from build123d import *

# Parameters (mm, degrees)
SKETCH1_R           = 21
SKETCH1_R_2         = 6
BOSS_EXTRUDE1_DEPTH = 1
SKETCH2_R           = 21
SKETCH2_R_2         = 2.7
SKETCH2_R_3         = 6
BOSS_EXTRUDE2_DEPTH = 5
SKETCH3_R           = 1.3
CUT_EXTRUDE1_DEPTH  = 4


with BuildPart() as part:
    # Sketch1 → Boss-Extrude1 (new body)
    with BuildSketch(Plane(origin=(0, 0, 0), x_dir=(1, 0, 0), z_dir=(0, 1, 0))):
        with Locations(Location((0, 0, 0), (0, 0, 270))):
            Circle(SKETCH1_R)
        with Locations(Location((0, 0, 0), (0, 0, 270))):
            Circle(SKETCH1_R_2, mode=Mode.SUBTRACT)
    extrude(amount=BOSS_EXTRUDE1_DEPTH)

    # Sketch2 → Boss-Extrude2 (add)
    with BuildSketch(Plane(origin=(0, 1, 0), x_dir=(1, 0, 0), z_dir=(0, 1, 0))):
        with Locations(Location((0, 0, 0), (0, 0, 270))):
            Circle(SKETCH2_R)
        with Locations(Location((0, 17, 0), (0, 0, 270))):
            Circle(SKETCH2_R_2, mode=Mode.SUBTRACT)
        with Locations(Location((14.722431864, -8.5, 0), (0, 0, 270))):
            Circle(SKETCH2_R_2, mode=Mode.SUBTRACT)
        with Locations(Location((-14.722431864, -8.5, 0), (0, 0, 270))):
            Circle(SKETCH2_R_2, mode=Mode.SUBTRACT)
        with Locations(Location((0, 0, 0), (0, 0, 270))):
            Circle(SKETCH2_R_3, mode=Mode.SUBTRACT)
        with BuildLine():
            Line((-0.75, 12.316251501), (-0.75, 8.31790238))
            ThreePointArc((-0.75, 8.31790238), (-0.97350713, 7.687776342), (-1.544117647, 7.339325629))
            ThreePointArc((-1.544117647, 7.339325629), (-6.495190528, 3.75), (-7.128101265, -2.332417706))
            ThreePointArc((-7.128101265, -2.332417706), (-7.144563176, -3.000806265), (-7.578514767, -3.509432137))
            Line((-7.578514767, -3.509432137), (-11.041186679, -5.508606698))
            ThreePointArc((-11.041186679, -5.508606698), (-11.624105203, -5.639137624), (-12.177435716, -5.414065035))
            ThreePointArc((-12.177435716, -5.414065035), (-14.508194092, -4.505741348), (-16.922739342, -5.159543893))
            ThreePointArc((-16.922739342, -5.159543893), (-17.83709693, -5.255719057), (-18.443528223, -4.564675969))
            ThreePointArc((-18.443528223, -4.564675969), (-16.454482672, 9.5), (-5.268638762, 18.254901961))
            ThreePointArc((-5.268638762, 18.254901961), (-4.366962246, 18.075238599), (-3.993073588, 17.235294118))
            ThreePointArc((-3.993073588, 17.235294118), (-3.352010576, 14.817335321), (-1.4, 13.253001201))
            ThreePointArc((-1.4, 13.253001201), (-0.928416164, 12.886339214), (-0.75, 12.316251501))
        make_face(mode=Mode.SUBTRACT)
        with BuildLine():
            Line((0.75, 12.316251501), (0.75, 8.31790238))
            ThreePointArc((0.75, 8.31790238), (0.97350713, 7.687776342), (1.544117647, 7.339325629))
            ThreePointArc((1.544117647, 7.339325629), (6.495190528, 3.75), (7.128101265, -2.332417706))
            ThreePointArc((7.128101265, -2.332417706), (7.144563176, -3.000806265), (7.578514767, -3.509432137))
            Line((7.578514767, -3.509432137), (11.041186679, -5.508606698))
            ThreePointArc((11.041186679, -5.508606698), (11.624105203, -5.639137624), (12.177435716, -5.414065035))
            ThreePointArc((12.177435716, -5.414065035), (14.508194092, -4.505741348), (16.922739342, -5.159543893))
            ThreePointArc((16.922739342, -5.159543893), (17.83709693, -5.255719057), (18.443528223, -4.564675969))
            ThreePointArc((18.443528223, -4.564675969), (16.454482672, 9.5), (5.268638762, 18.254901961))
            ThreePointArc((5.268638762, 18.254901961), (4.366962246, 18.075238599), (3.993073588, 17.235294118))
            ThreePointArc((3.993073588, 17.235294118), (3.352010576, 14.817335321), (1.4, 13.253001201))
            ThreePointArc((1.4, 13.253001201), (0.928416164, 12.886339214), (0.75, 12.316251501))
        make_face(mode=Mode.SUBTRACT)
        with BuildLine():
            Line((10.291186679, -6.807644803), (6.828514767, -4.808470243))
            ThreePointArc((6.828514767, -4.808470243), (6.171056046, -4.686970077), (5.583983618, -5.006907923))
            ThreePointArc((5.583983618, -5.006907923), (0, -7.5), (-5.583983618, -5.006907923))
            ThreePointArc((-5.583983618, -5.006907923), (-6.171056046, -4.686970077), (-6.828514767, -4.808470243))
            Line((-6.828514767, -4.808470243), (-10.291186679, -6.807644803))
            ThreePointArc((-10.291186679, -6.807644803), (-10.695689039, -7.24720159), (-10.777435716, -7.838936166))
            ThreePointArc((-10.777435716, -7.838936166), (-11.156183517, -10.311593973), (-12.929665754, -12.075750225))
            ThreePointArc((-12.929665754, -12.075750225), (-13.470134683, -12.819519543), (-13.174889461, -13.690225991))
            ThreePointArc((-13.174889461, -13.690225991), (0, -19), (13.174889461, -13.690225991))
            ThreePointArc((13.174889461, -13.690225991), (13.470134683, -12.819519543), (12.929665754, -12.075750225))
            ThreePointArc((12.929665754, -12.075750225), (11.156183517, -10.311593973), (10.777435716, -7.838936166))
            ThreePointArc((10.777435716, -7.838936166), (10.695689039, -7.24720159), (10.291186679, -6.807644803))
        make_face(mode=Mode.SUBTRACT)
    extrude(amount=BOSS_EXTRUDE2_DEPTH)

    # Sketch3 → Cut-Extrude1 (cut)
    with BuildSketch(Plane(origin=(0, 1, 0), x_dir=(1, 0, 0), z_dir=(0, 1, 0))):
        with Locations(Location((-14.722431864, -8.5, 0), (0, 0, 270))):
            Circle(SKETCH3_R)
        with Locations(Location((14.722431864, -8.5, 0), (0, 0, 270))):
            Circle(SKETCH3_R)
        with Locations(Location((0, 17, 0), (0, 0, 270))):
            Circle(SKETCH3_R)
    extrude(amount=-CUT_EXTRUDE1_DEPTH, mode=Mode.SUBTRACT)


solid = part.part
Geometry check sheet. Reference: the model listing, model coordinates, mm. A direction names the side the tool comes from. Coordinates: 2 decimals unless noted, no trailing zeros. Order: outer loops, then holes, each group sorted by start corner. A loop starts at its lowest first (then second) coordinate and runs counter-clockwise, first axis right, second up. Notation, with made-up numbers: (-4.5, 55) -> (52.5, 55) arc R18 ccw to (52.5, 86) -> close; hole circle Ø5 at (49.25, -30). An arc over 180 degrees is marked (long way). Use a Markdown table: item, result. Add a question column.
1. Cross-section at D-D (z = 13). Enter the section's corners in (x, y), and give its area (3 significant figures).
2. Material ranges on L1, parallel to Z at x = -14, y = 1.3; L2, parallel to X at y = 4.6, z = 9; L3, parallel to Z at x = -4.5, y = 5.35, recorded low to high.
3. Go/stop test with flat-tipped pins: pin 1 Ø1 at (y, z) = (4, 16.5) entering from +X; pin 2 Ø5 at (x, z) = (-14.72, 8.5) entering from +Y; pin 3 Ø3 at (y, z) = (2.5, -11.5) entering from +X. Record where each tip stops, or that it passes through.
4. Set-up check for faces 5 (the face through (1.802, 2.958, 5.723)), 6 (the face through (-0.75, 3, -10)): record each of +Z, -Z, +X, -X, +Y, -Y from which the full face is reachable in a straight line by a thin tool's end or side.
5. Mould release check, pull along Z, two halves, no side actions. Record for faces 1 (the face through (-13.47, 3.46, 12.81)), 2 (the face through (0.75, 3, -10)), 3 (the face through (-4.4, 0, 4.4)), 4 (the face through (6.31, 2.96, 20.03)): pulls with the +Z half, pulls with the -Z half, needs draft (parallel to the pull), parting line crosses it, or undercut.
6. Cross-section at B-B (z = 8.5). Enter the section's corners in (x, y).
7. Cross-section at A-A (z = 0). Enter the section's corners in (x, y), and give its area (3 significant figures).
8. Cross-section at C-C (x = 9). Enter the section's corners in (y, z), and give its area (3 significant figures).
Filled sheet:
| question | item | result |
|---|---|---|
| 1 | outline | (-16.49, 0) -> (16.49, 0) -> (16.49, 6) -> (13.48, 6) -> (13.48, 1) -> (-13.48, 1) -> (-13.48, 6) -> (-16.49, 6) -> close |
| 1 | area | 63.1 mm2 |
| 2 | L1 | -15.65 to -12.85, 4.57 to 5.9, 11.1 to 15.65 |
| 2 | L2 | -18.97 to -17.38, -12.07 to -10.75, 10.75 to 12.07, 17.38 to 18.97 |
| 2 | L3 | -20.51 to -18.17, -6 to -3.97, 3.97 to 6, 18.46 to 20.51 |
| 3 | pin 1 | x = 13.6 |
| 3 | pin 2 | y = 1 |
| 3 | pin 3 | x = 18.47 |
| 4 | face 5 | +Y, -Y |
| 4 | face 6 | +Y |
| 5 | face 1 | undercut |
| 5 | face 2 | undercut |
| 5 | face 3 | needs draft |
| 5 | face 4 | parting line crosses it |
| 6 | outline | (-19.2, 0) -> (-16.02, 0) -> (-16.02, 1) -> (-17.42, 1) -> (-17.42, 6) -> (-19.2, 6) -> close; (-13.42, 0) -> (13.42, 0) -> (13.42, 1) -> (12.02, 1) -> (12.02, 6) -> (10.72, 6) -> (10.72, 1) -> (-10.72, 1) -> (-10.72, 6) -> (-12.02, 6) -> (-12.02, 1) -> (-13.42, 1) -> close; (16.02, 0) -> (19.2, 0) -> (19.2, 6) -> (17.42, 6) -> (17.42, 1) -> (16.02, 1) -> close |
| 7 | outline | (-21, 0) -> (-6, 0) -> (-6, 6) -> (-7.5, 6) -> (-7.5, 1) -> (-19, 1) -> (-19, 6) -> (-21, 6) -> close; (6, 0) -> (21, 0) -> (21, 6) -> (19, 6) -> (19, 1) -> (7.5, 1) -> (7.5, 6) -> (6, 6) -> close |
| 7 | area | 65.0 mm2 |
| 8 | outline | (0, -18.97) -> (6, -18.97) -> (6, -16.73) -> (1, -16.73) -> (1, 4.33) -> (6, 4.33) -> (6, 6.06) -> (1, 6.06) -> (1, 16.73) -> (6, 16.73) -> (6, 18.97) -> (0, 18.97) -> close |
| 8 | area | 69.0 mm2 |
